```python
from build123d import *

# Parameters (mm, degrees)
BOSS_EXTRUDE1_DEPTH = 50
SHELL2_START        = 2
SHELL2_DEPTH        = 48


# Read off the part's stored shape, not the designer's step: Shell2
with BuildPart() as part:
    # Sketch1 → Boss-Extrude1 (new body)
    with BuildSketch(Plane(origin=(0, 0, 0), x_dir=(1, 0, 0), z_dir=(0, 1, 0))):
        with BuildLine():
            Line((-26.477298014, 20.407046949), (26.477298014, 20.407046949))
            ThreePointArc((26.477298014, 20.407046949), (46.884344963, 0), (26.477298014, -20.407046949))
            Line((26.477298014, -20.407046949), (-26.477298014, -20.407046949))
            ThreePointArc((-26.477298014, -20.407046949), (-46.884344963, 0), (-26.477298014, 20.407046949))
        make_face()
    extrude(amount=BOSS_EXTRUDE1_DEPTH)

    # Shell2 outline → Shell2 (cut)
    with BuildSketch(Plane(origin=(0, 0, 0), x_dir=(1, 0, 0), z_dir=(0, 1, 0)).offset(SHELL2_START)):
        with BuildLine():
            Line((-26.477298014, -18.407046949), (-26.477298014, -20.407046949))
            Line((-26.477298014, -20.407046949), (26.477298014, -20.407046949))
            Line((26.477298014, -20.407046949), (26.477298014, -18.407046949))
            ThreePointArc((26.477298014, -18.407046949), (44.884344963, 0), (26.477298014, 18.407046949))
            Line((26.477298014, 18.407046949), (-26.477298014, 18.407046949))
            ThreePointArc((-26.477298014, 18.407046949), (-44.884344963, 0), (-26.477298014, -18.407046949))
        make_face()
    extrude(amount=SHELL2_DEPTH, mode=Mode.SUBTRACT)


solid = part.part
```
Design review of the part built by this model. Coordinates are the model's own, in mm. A direction names the side the tool comes from. Give positions to 0.01 mm unless a question says otherwise; leave off trailing zeros. Loops run counter-clockwise (first coordinate to the right, second up) from the corner with the lowest first, then second, coordinate; pieces in that order, holes last. Notation, with made-up numbers: (19, 15.5) -> (46, 15.5) arc R31 ccw to (46, 41.5) -> close; hole circle Ø2 at (-17.5, 28). An arc over 180 degrees is marked (long way). One line per item, written item: value.
Q1. For L1, parallel to Z at x = -24, y = 6.5; L2, parallel to Y at x = 21, z = -1.5; L3, parallel to X at y = 34.5, z = -1.5, list the stretches that pass through material, from the lowest coordinate up.
Numbers:
L1: z = -20.41 to -18.41
L2: y = 0 to 2
L3: x = -46.83 to -44.82, 44.82 to 46.83
Q2. We need section C-C on z = 0. Give the boundary of the cut face in (x, y), and give its area (3 significant figures).
Numbers:
outline: (-46.88, 0) -> (46.88, 0) -> (46.88, 50) -> (44.88, 50) -> (44.88, 2) -> (-44.88, 2) -> (-44.88, 50) -> (-46.88, 50) -> close
area: 380 mm^2
Q3. Machinability: for faces 4 (the cylindrical face through (46.88, 24.65, -0.45)), 5 (the cylindrical face through (44.88, 25.66, 0.4)), 6 (the flat face through (26.477, 26, 19)), which of the approach directions +Z, -Z, +X, -X, +Y, -Y give a long, thin tool a straight path to every point of the face, cutting with its end or side? Answer none if there is none.
Numbers:
face 4: +X, +Y, -Y
face 5: +Y
face 6: +Z, +Y
Q4. For pin 1 Ø6 at (y, z) = (25.5, -1.5) entering from -X; pin 2 Ø1.6 at (y, z) = (19, 19) entering from +X; pin 3 Ø5 at (x, y) = (-14.5, 40.5) entering from +Z; pin 4 Ø3 at (x, z) = (-20, -8.5) entering from -Y, all flat-tipped, find the tip position at first contact; note any pin that passes through.
Numbers:
pin 1: stops at x = -46.88
pin 2: stops at x = 35.71
pin 3: stops at z = -18.41
pin 4: stops at y = 0
Q5. Draft analysis for pull direction Z (two halves, no side actions). For faces 1 (the cylindrical face through (-46.88, 24.65, 0.45)), 2 (the cylindrical face through (-44.88, 25.66, -0.4)), 3 (the flat face through (1, 0, 0)), state which applies: pulls with the +Z half, pulls with the -Z half, needs draft (parallel to the pull), parting line crosses it, or undercut.
Numbers:
face 1: parting line crosses it
face 2: undercut
face 3: needs draft
Q6. We need section A-A on y = 29. Give the boundary of the cut face in (x, z).
Numbers:
outline: (-26.48, -20.41) -> (26.48, -20.41) arc R20.41 ccw to (26.48, 20.41) -> (26.48, 18.41) arc R18.41 cw to (26.48, -18.41) -> (-26.48, -18.41) arc R18.41 cw to (-26.48, 18.41) -> (-26.48, 20.41) arc R20.41 ccw to start
Q7. We need section B-B on x = 20.5. Give the boundary of the cut face in (y, z).
Numbers:
outline: (0, -20.41) -> (50, -20.41) -> (50, -18.41) -> (2, -18.41) -> (2, 20.41) -> (0, 20.41) -> close
